Autodesk Inventor part; units mm, degrees
ref_plane "Work Plane1" through (0.475, -40, 0) normal (1, 0, 0) x (0, 0, -1)
ref_plane "YZ Plane" through (0, 0, 0) normal (1, 0, 0) x (0, 1, 0)
ref_plane "XZ Plane" through (0, 0, 0) normal (0, 1, 0) x (-1, 0, 0)
sketch "Sketch1" plane through (0, 0, 0) normal (0, 0, 1) x (1, 0, 0)
  line L0 (-59.525, 40) -> (60.475, 40)
  line L1 (60.475, 40) -> (60.475, -40)
  line L2 (60.475, -40) -> (-59.525, -40)
  line L3 (-59.525, -40) -> (-59.525, 40)
  line L4 (-59.525, 40) -> (60.475, -40) construction
  line L5 (60.475, 40) -> (-59.525, -40) construction
  line L6 (-34.525, -65) -> (-34.525, 60.8703) construction
  line L7 (50.475, -61.0061) -> (50.475, 64.8642) construction
  line L8 (-67.2304, -35) -> (77.4738, -35) construction
  line L9 (-68.2264, 35) -> (76.4779, 35) construction
  line L10 (-2.025, -66.0646) -> (-2.025, 59.8057) construction
  line L11 (2.975, -64.9269) -> (2.975, 60.9434) construction
  line L12 (-67.6256, -30) -> (77.0786, -30) construction
  line L13 (-69.0671, 30) -> (75.6371, 30) construction
  line L14 (55.475, -60.5874) -> (55.475, 65.2829) construction
  line L15 (-54.525, -62.7211) -> (-54.525, 63.1492) construction
  line L16 (-55.475, -32.5) -> (-53.575, -32.5)
  line L17 (-53.575, -32.5) -> (-53.575, -27.5)
  line L18 (-53.575, -27.5) -> (-55.475, -27.5)
  line L19 (-55.475, -27.5) -> (-55.475, -32.5)
  line L20 (-55.475, -32.5) -> (-53.575, -27.5) construction
  line L21 (-53.575, -32.5) -> (-55.475, -27.5) construction
  line L22 (56.425, -32.5) -> (54.525, -32.5)
  line L23 (54.525, -32.5) -> (54.525, -27.5)
  line L24 (54.525, -27.5) -> (56.425, -27.5)
  line L25 (56.425, -27.5) -> (56.425, -32.5)
  line L26 (56.425, -32.5) -> (54.525, -27.5) construction
  line L27 (54.525, -32.5) -> (56.425, -27.5) construction
  line L28 (-53.575, 32.5) -> (-55.475, 32.5)
  line L29 (-55.475, 32.5) -> (-55.475, 27.5)
  line L30 (-55.475, 27.5) -> (-53.575, 27.5)
  line L31 (-53.575, 27.5) -> (-53.575, 32.5)
  line L32 (-53.575, 32.5) -> (-55.475, 27.5) construction
  line L33 (-55.475, 32.5) -> (-53.575, 27.5) construction
  line L34 (56.425, 32.5) -> (54.525, 32.5)
  line L35 (54.525, 32.5) -> (54.525, 27.5)
  line L36 (54.525, 27.5) -> (56.425, 27.5)
  line L37 (56.425, 27.5) -> (56.425, 32.5)
  line L38 (56.425, 32.5) -> (54.525, 27.5) construction
  line L39 (54.525, 32.5) -> (56.425, 27.5) construction
  line L40 (-34.525, 35) -> (50.475, 35)
  line L41 (50.475, 35) -> (50.475, -35)
  line L42 (50.475, -35) -> (-34.525, -35)
  line L43 (-34.525, -35) -> (-34.525, 35)
  point P0 (0.475, 0)
  point P1 (-2.025, 35)
  point P2 (2.975, -35)
  point P3 (50.475, 35)
  point P4 (55.475, 36)
  point P5 (56, 37)
  point P6 (-54.525, -30)
  point P7 (55.475, -30)
  point P8 (-54.525, 30)
  point P9 (55.475, 30)
  dimension "d0" = 120
  dimension "d1" = 80
  dimension "d9" = 25
  dimension "d10" = 10
  dimension "d11" = 5
  dimension "d12" = 5
  dimension "d20" = 10
  dimension "d21" = 10
  dimension "d22" = 5
  dimension "d23" = 5
  dimension "d26" = 1.9
  dimension "d27" = 5
  dimension "d28" = 1.9
  dimension "d29" = 1.9
  dimension "d30" = 5
  dimension "d31" = 1.9
extrude "Extrusion1" add sketch "Sketch1" along normal blind 4 contours L0 L1 L2 L3 | L19 L18 L17 L16 | L22 L23 L24 L25 | L31 L30 L29 L28 | L37 L36 L35 L34 | L40 L41 L42 L43
sketch "Sketch2" plane through (60.475, -40, 0) normal (1, 0, 0) x (0, 0, -1)
  line L0 (0, 40) -> (-8.8455, 40) construction
  line L1 (-2, -5.0193) -> (-2, 56.2537) construction
  line L2 (-4, 0) -> (-4, 80) construction
  line L3 (1.2244, 10) -> (-7.6211, 10) construction
  line L4 (0, 0) -> (-4, 0) construction
  circle A0 centre (-2, 10) radius 1.25
  circle A1 centre (-2, 70) radius 1.25
  dimension "d4" = 2
  dimension "d5" = 10
  dimension "d6" = 2.5
extrude "Extrusion3" cut sketch "Sketch2" against normal blind 20
extrude "Extrusion4" cut sketch "Sketch1" along normal blind 10 contours L19 L18 L17 L16 | L22 L23 L24 L25 | L31 L30 L29 L28 | L37 L36 L35 L34
ref_plane "Work Plane1" through (0.475, -40, 0) normal (1, 0, 0) x (0, 0, -1)
mirror "Mirror1" about plane through (0.475, -40, 0) normal (1, 0, 0) of "Extrusion3"
extrude "Extrusion6" cut sketch "Sketch1" along normal blind 10 contours L40 L41 L42 L43
sketch "Sketch3" plane through (0, 0, 4) normal (0, 0, 1) x (1, 0, 0)
  line L0 (0, 0) -> (-78.4813, 0) construction
  line L1 (-44.525, 48.1643) -> (-44.525, -53.6198) construction
  line L2 (-34.525, -35) -> (-34.525, 35) construction
  line L3 (-48.525, 23.5) -> (-40.525, 23.5)
  line L4 (-40.525, 23.5) -> (-40.525, 10)
  line L5 (-40.525, 10) -> (-48.525, 10)
  line L6 (-48.525, 10) -> (-48.525, 23.5)
  line L7 (-53.525, 48.2216) -> (-53.525, -53.5625) construction
  circle A0 centre (-53.525, 20.95) radius 2.55
  circle A1 centre (-53.525, 12.55) radius 2.55
  line L8 (-47.3423, 23.5) -> (-70.4402, 23.5) construction
  line L9 (-47.3423, 10) -> (-69.2245, 10) construction
  line L10 (60.475, 40) -> (-59.525, 40)
  point P0 (-44.525, 0)
  point P1 (-53.525, 1)
  dimension "d38" = 10
  dimension "d39" = 8
  dimension "d40" = 13.5
  dimension "d41" = 5
  dimension "d42" = 5.1
  dimension "d43" = 5.1
  dimension "d47" = 30
extrude "Extrusion7" cut sketch "Sketch3" against normal blind 10
sketch "Sketch5" plane through (0, 0, 0) normal (0, 0, -1) x (-1, 0, 0)
  line L0 (48.525, 10) -> (40.525, 10) construction
  line L1 (40.525, 10) -> (40.525, 23.5) construction
  line L2 (40.525, 23.5) -> (48.525, 23.5) construction
  line L3 (48.525, 23.5) -> (48.525, 10) construction
  line L4 (48.525, 10) -> (40.525, 10) construction
  line L5 (48.525, 23.5) -> (48.525, 10) construction
  line L6 (49.525, 9) -> (39.525, 9)
  line L7 (39.525, 9) -> (39.525, 24.5)
  line L8 (39.525, 24.5) -> (49.525, 24.5)
  line L9 (49.525, 24.5) -> (49.525, 9)
  point P0 (0, 0)
  dimension "d48" = 1
extrude "Extrusion8" cut sketch "Sketch5" against normal blind 3
properties part number "Topshelf"
Geometry check sheet. Reference: the model listing, model coordinates, mm. A direction names the side the tool comes from. Round coordinates to 2 decimals unless told otherwise and drop trailing zeros. Loops run counter-clockwise (first coordinate to the right, second up) from the corner with the lowest first, then second, coordinate; pieces in that order, holes last.
Item 1: Mould release check, pull along Y, two halves, no side actions. Record for faces 1 (the flat face through (-55.475, -30, 0.6)), 2 (the flat face through (-59.525, -1, 2)): pulls with the +Y half, pulls with the -Y half, needs draft (parallel to the pull), parting line crosses it, or undercut.
Item 2: Thickness scan on line 1 (X direction, y = 15.5, z = 0.25) (3 decimals); line 2 (Y direction, x = 57.8, z = 2); line 3 (X direction, y = -27, z = 2) (3 decimals). Record the ranges inside material, lowest first.
Item 3: Cross-section at D-D on y = -30. Count the separate pieces of the cut face and the enclosed holes in it, then the cut area to 3 significant figures.
Item 4: Gauge pin test, flat ends, axial feed: pin 1 (1.2 mm diameter, centred on y = -31, z = 2.5, fed in from +X) (3 decimals); pin 2 (1.5 mm diameter, centred on x = -46.5, y = 19, fed in from -Z). Record the tip position at first contact, or that the pin passes through.
Item 5: Access from +Z, -Z, +X, -X, +Y, -Y to the whole of each face (thin tool, end or side, straight path). Record for faces 3 (the cylindrical face through (-46.648, 28.946, 1.328)), 4 (the cylindrical face through (58.48, 30.38, 0.81)), 5 (the flat face through (-53.575, -30, 0.6)), 6 (the flat face through (-44, 24.5, 1)).
Item 6: Cross-section at B-B on y = 20.95. Record the boundary of the cut face in (x, z) (3 decimals).
Item 7: Cross-section at C-C on y = 6. Record the boundary of the cut face in (x, z) (3 decimals).
Item 8: Cross-section at A-A on x = -12. Record the boundary of the cut face in (y, z).
Answer sheet:
1. face 1: undercut
1. face 2: needs draft
2. line 1: x = -59.525 to -49.525, -39.525 to -34.525, 50.475 to 60.475
2. line 2: y = -40 to -31.25, -28.75 to 28.75, 31.25 to 40
2. line 3: x = -59.525 to -34.525, 50.475 to 60.475
3. separate pieces: 7
3. enclosed holes: 0
3. area: 59.3 mm2
4. pin 1: stops at x = 60.475
4. pin 2: passes through
5. face 3: -X
5. face 4: +X
5. face 5: +Z, -Z
5. face 6: -Z
6. outline: (-59.525, 0) - (-56.075, 0) - (-56.075, 4) - (-59.525, 4) - close; (-50.975, 0) - (-49.525, 0) - (-49.525, 3) - (-48.525, 3) - (-48.525, 4) - (-50.975, 4) - close; (-40.525, 3) - (-39.525, 3) - (-39.525, 0) - (-34.525, 0) - (-34.525, 4) - (-40.525, 4) - close; (50.475, 0) - (60.475, 0) - (60.475, 4) - (50.475, 4) - close
7. outline: (-59.525, 0) - (-34.525, 0) - (-34.525, 4) - (-59.525, 4) - close; (50.475, 0) - (60.475, 0) - (60.475, 4) - (50.475, 4) - close
8. outline: (-40, 0) - (-35, 0) - (-35, 4) - (-40, 4) - close; (35, 0) - (40, 0) - (40, 4) - (35, 4) - close
